```python
from build123d import *

# Parameters (mm, degrees)
SKETCH1_R           = 2
SKETCH1_R_2         = 1.65
BOSS_EXTRUDE1_DEPTH = 4.5


with BuildPart() as part:
    # Sketch1 → Boss-Extrude1 (new body)
    with BuildSketch(Plane(origin=(0, 4.5, 0), x_dir=(1, 0, 0), z_dir=(0, 1, 0))):
        with BuildLine():
            Line((5.5, 12), (-5.5, 12))
            ThreePointArc((-5.5, 12), (-6.914213562, 11.414213562), (-7.5, 10))
            Line((-7.5, 10), (-7.5, -10))
            ThreePointArc((-7.5, -10), (-6.914213562, -11.414213562), (-5.5, -12))
            Line((-5.5, -12), (5.5, -12))
            ThreePointArc((5.5, -12), (6.914213562, -11.414213562), (7.5, -10))
            Line((7.5, -10), (7.5, 10))
            ThreePointArc((7.5, 10), (6.914213562, 11.414213562), (5.5, 12))
        make_face()
        Circle(SKETCH1_R, mode=Mode.SUBTRACT)
        with Locations((0, -8)):
            Circle(SKETCH1_R_2, mode=Mode.SUBTRACT)
        with Locations((0, 8)):
            Circle(SKETCH1_R_2, mode=Mode.SUBTRACT)
    extrude(amount=-BOSS_EXTRUDE1_DEPTH)


solid = part.part
```
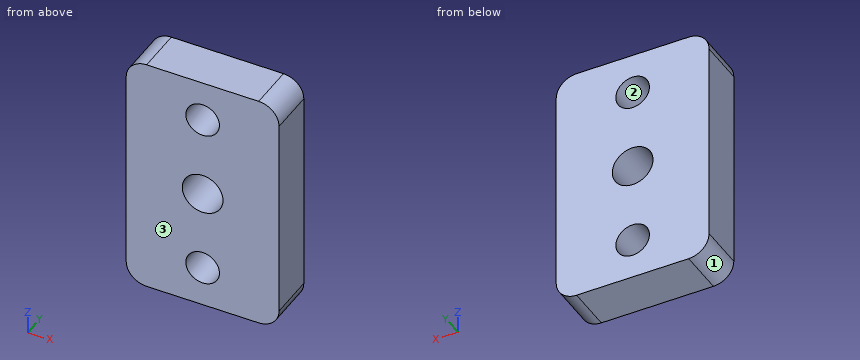
Model file for the job. Use its own axes, mm. Face numbers are marked on the shaded views. Round coordinates to 2 decimals unless told otherwise and drop trailing zeros. Order: outer loops, then holes, each group sorted by start corner. A loop starts at its lowest first (then second) coordinate and runs counter-clockwise, first axis right, second up. Notation, with made-up numbers: (67.5, 67.25) -> (104.5, 67.25) arc R14 cw to (104.5, 85.25) -> close; hole circle Ø10 at (88, 21). An arc over 180 degrees is marked (long way). Use one line per item in the form item = value.
Item 1: Cut at A-A, the plane z = 8. Write the cut outline in (x, y).
Returned:
outline = (-7.5, 0) -> (-1.65, 0) -> (-1.65, 4.5) -> (-7.5, 4.5) -> close; (1.65, 0) -> (7.5, 0) -> (7.5, 4.5) -> (1.65, 4.5) -> close
Item 2: Cut at C-C, the plane y = 2.3. Write the cut outline in (x, z).
Returned:
outline = (-7.5, -10) arc R2 ccw to (-5.5, -12) -> (5.5, -12) arc R2 ccw to (7.5, -10) -> (7.5, 10) arc R2 ccw to (5.5, 12) -> (-5.5, 12) arc R2 ccw to (-7.5, 10) -> close; hole circle Ø4 at (0, 0); hole circle Ø3.3 at (0, -8); hole circle Ø3.3 at (0, 8)
Item 3: Pull direction X, two halves, no side cores. Call the marked faces 1, 2 and 3: released by +X, released by -X, zero draft, split by the parting line, or undercut.
Returned:
face_1 = released by -X
face_2 = undercut
face_3 = zero draft
Item 4: Flat gauge pins, fed straight in: pin 1 Ø6 at (x, z) = (4, 7.5) entering from -Y; pin 2 Ø3 at (x, z) = (0, 8) entering from +Y. Where does each tip first touch, or does it go through?
Returned:
pin_1 = 0
pin_2 = through
Item 5: Cut at B-B, the plane x = 0. Write the cut outline in (y, z).
Returned:
outline = (0, -12) -> (4.5, -12) -> (4.5, -9.65) -> (0, -9.65) -> close; (0, -6.35) -> (4.5, -6.35) -> (4.5, -2) -> (0, -2) -> close; (0, 2) -> (4.5, 2) -> (4.5, 6.35) -> (0, 6.35) -> close; (0, 9.65) -> (4.5, 9.65) -> (4.5, 12) -> (0, 12) -> close
Item 6: Drill centre lines: line 1 (Z direction, x = 0, y = 2.3); line 2 (X direction, y = 1, z = -8); line 3 (Z direction, x = 0.5, y = 2.15). Where is each one in solid material? Low to high.
Returned:
line_1 = -12 to -9.65, -6.35 to -2, 2 to 6.35, 9.65 to 12
line_2 = -7.5 to -1.65, 1.65 to 7.5
line_3 = -12 to -9.57, -6.43 to -1.94, 1.94 to 6.43, 9.57 to 12
Item 7: Cut at D-D, the plane z = 0. Write the cut outline in (x, y), and give its area (3 significant figures).
Returned:
outline = (-7.5, 0) -> (-2, 0) -> (-2, 4.5) -> (-7.5, 4.5) -> close; (2, 0) -> (7.5, 0) -> (7.5, 4.5) -> (2, 4.5) -> close
area = 49.5 mm^2
